Could you check a few things on this model? Use its own coordinates, in mm. A direction names the side the tool comes from. Round coordinates to 2 decimals unless told otherwise and drop trailing zeros. Write each loop counter-clockwise with the first axis right and the second up, starting at its lowest first coordinate (ties: lowest second). Pieces come first, ordered by that corner, then holes. Notation, with made-up numbers: (62, 65.25) - (87, 65.25) arc R34 cw to (87, 96.25) - close; hole circle Ø6 at (34, 36.5). An arc over 180 degrees is marked (long way). Write each question's results on one line, items separated by ' | '. Start each with the question number.
(1) Imagine slicing it at D-D on x = 56.5. Write out the boundary of the cut face in (y, z), then the cut area to 3 significant figures.
(2) For P1, Ø10, axis at x = 58.5, y = 25, coming from the +Z side; P2, Ø12, axis at y = 13.5, z = -13, coming from the -X side; P3, Ø5.5, axis at x = -12.5, z = 76.5, coming from the -Y side; P4, Ø4.5, axis at x = -78.46, z = -15.2, coming from the +Y side, each with a flat end and sliding along its axis, tell me the tip position at first contact or that it passes through.
(3) Please list where these lines run through material, in increasing order: line 1 (Y direction, x = 46, z = -25); line 2 (X direction, y = 28, z = 8); line 3 (Z direction, x = 58, y = 20). Write a range as [from, to].
(4) Imagine slicing it at A-A on x = 1. Write out the boundary of the cut face in (y, z).
(5) Imagine slicing it at C-C on x = -24.13. Write out the boundary of the cut face in (y, z).
(6) On a 3-axis mill with a long thin cutter (end or side, diameter ignored), from which of +Z, -Z, +X, -X, +Y, -Y can I reach the whole of each face in a straight line? I mean faces 1 (the flat face through (62, 20, 8.771)), 2 (the flat face through (69.3, 20, 1)), 3 (the flat face through (21.14, 2, 6)), 4 (the flat face through (62, 20, -6.229)), 5 (the flat face through (54.3, 20, 1)). Say none if no direction works.
(7) Imagine slicing it at B-B on z = 11. Write out the boundary of the cut face in (x, y).
```python
from build123d import *

# Parameters (mm, degrees)
SKETCH1_W           = 170
SKETCH1_H           = 158
SKETCH1_R           = 1.75
SKETCH1_R_2         = 2.55
SKETCH1_W_2         = 42.27
SKETCH1_H_2         = 22
BOSS_EXTRUDE1_DEPTH = 5
SKETCH2_W           = 15
SKETCH2_H           = 15
BOSS_EXTRUDE2_DEPTH = 30


with BuildPart() as part:
    # Sketch1 → Boss-Extrude1 (new body)
    with BuildSketch(Plane(origin=(0, 0, 0), x_dir=(1, 0, 0), z_dir=(0, 1, 0))):
        Rectangle(SKETCH1_W, SKETCH1_H)
        with Locations(Location((82.5, 76.5, 0), (0, 0, 270))):
            Circle(SKETCH1_R, mode=Mode.SUBTRACT)
        with Locations(Location((22.5, 76.5, 0), (0, 0, 270))):
            Circle(SKETCH1_R, mode=Mode.SUBTRACT)
        with Locations(Location((5, 76.5, 0), (0, 0, 270))):
            Circle(SKETCH1_R, mode=Mode.SUBTRACT)
        with Locations(Location((-12.5, 76.5, 0), (0, 0, 270))):
            Circle(SKETCH1_R, mode=Mode.SUBTRACT)
        with Locations(Location((-30, 76.5, 0), (0, 0, 270))):
            Circle(SKETCH1_R, mode=Mode.SUBTRACT)
        with Locations(Location((-47.5, 76.5, 0), (0, 0, 270))):
            Circle(SKETCH1_R, mode=Mode.SUBTRACT)
        with Locations(Location((82.5, -76.5, 0), (0, 0, 270))):
            Circle(SKETCH1_R, mode=Mode.SUBTRACT)
        with Locations(Location((22.5, -76.5, 0), (0, 0, 270))):
            Circle(SKETCH1_R, mode=Mode.SUBTRACT)
        with Locations(Location((5, -76.5, 0), (0, 0, 270))):
            Circle(SKETCH1_R, mode=Mode.SUBTRACT)
        with Locations(Location((-12.5, -76.5, 0), (0, 0, 270))):
            Circle(SKETCH1_R, mode=Mode.SUBTRACT)
        with Locations(Location((-30, -76.5, 0), (0, 0, 270))):
            Circle(SKETCH1_R, mode=Mode.SUBTRACT)
        with Locations(Location((-47.5, -76.5, 0), (0, 0, 270))):
            Circle(SKETCH1_R, mode=Mode.SUBTRACT)
        with Locations(Location((80, 15.2, 0), (0, 0, 270))):
            Circle(SKETCH1_R, mode=Mode.SUBTRACT)
        with Locations(Location((-78.46, 15.2, 0), (0, 0, 270))):
            Circle(SKETCH1_R, mode=Mode.SUBTRACT)
        with Locations(Location((24.14, -11, 0), (0, 0, 270))):
            Circle(SKETCH1_R_2, mode=Mode.SUBTRACT)
        with Locations(Location((24.14, 0, 0), (0, 0, 270))):
            Circle(SKETCH1_R_2, mode=Mode.SUBTRACT)
        with Locations(Location((-24.13, 0, 0), (0, 0, 270))):
            Circle(SKETCH1_R_2, mode=Mode.SUBTRACT)
        with Locations(Location((-24.13, -11, 0), (0, 0, 270))):
            Circle(SKETCH1_R_2, mode=Mode.SUBTRACT)
        with Locations(Location((80, 65, 0), (0, 0, 270))):
            Circle(SKETCH1_R, mode=Mode.SUBTRACT)
        with Locations(Location((-78.46, 65, 0), (0, 0, 270))):
            Circle(SKETCH1_R, mode=Mode.SUBTRACT)
        with Locations(Location((76.811114527, -49.46471284, 0), (0, 0, 270))):
            Circle(SKETCH1_R, mode=Mode.SUBTRACT)
        with Locations(Location((27.541114527, -49.46471284, 0), (0, 0, 270))):
            Circle(SKETCH1_R, mode=Mode.SUBTRACT)
        with Locations((0.005, -5.5)):
            Rectangle(SKETCH1_W_2, SKETCH1_H_2, mode=Mode.SUBTRACT)
    extrude(amount=BOSS_EXTRUDE1_DEPTH)

    # Sketch2 → Boss-Extrude2 (add)
    with BuildSketch(Plane(origin=(0, 5, 0), x_dir=(1, 0, 0), z_dir=(0, 1, 0))):
        with Locations((61.800323829, -1.270769853)):
            Rectangle(SKETCH2_W, SKETCH2_H)
    extrude(amount=BOSS_EXTRUDE2_DEPTH)


solid = part.part
```
Response:
1) outline: (0, -79) - (5, -79) - (5, -6.23) - (35, -6.23) - (35, 8.77) - (5, 8.77) - (5, 79) - (0, 79) - close | area: 1,240 mm²
2) P1: z = 8.77 | P2: through | P3: y = 0 | P4: y = 5
3) line 1: [0, 5] | line 2: [54.3, 69.3] | line 3: [-6.23, 8.77]
4) outline: (0, -79) - (5, -79) - (5, -5.5) - (0, -5.5) - close; (0, 16.5) - (5, 16.5) - (5, 79) - (0, 79) - close
5) outline: (0, -79) - (5, -79) - (5, -2.55) - (0, -2.55) - close; (0, 2.55) - (5, 2.55) - (5, 8.45) - (0, 8.45) - close; (0, 13.55) - (5, 13.55) - (5, 79) - (0, 79) - close
6) face 1: +Z, +X, -X, +Y | face 2: +Z, -Z, +X, +Y | face 3: +Y, -Y | face 4: -Z, +X, -X, +Y | face 5: +Z, -Z, -X, +Y
7) outline: (-85, 0) - (-26.68, 0) - (-26.68, 5) - (-85, 5) - close; (-21.58, 0) - (-21.13, 0) - (-21.13, 5) - (-21.58, 5) - close; (21.14, 0) - (21.59, 0) - (21.59, 5) - (21.14, 5) - close; (26.69, 0) - (85, 0) - (85, 5) - (26.69, 5) - close
